Work out the finished part from the listing and answer in its coordinate system (mm). A direction names the side the tool comes from. Round coordinates to 2 decimals unless told otherwise and drop trailing zeros. Order: outer loops, then holes, each group sorted by start corner. A loop starts at its lowest first (then second) coordinate and runs counter-clockwise, first axis right, second up. Notation, with made-up numbers: (35.5, 21.5) - (64.5, 21.5) arc R24 ccw to (64.5, 46.5) - close; hole circle Ø4 at (-16, 33.25). An arc over 180 degrees is marked (long way). Use one line per item in the form item = value. Start each with the question number.
Q1. Which of the six approach directions +Z, -Z, +X, -X, +Y, -Y give full straight-line access (tool end or side, diameter ignored) to faces 1 (the cylindrical face through (77.496, 0.934, 0.986)), 2 (the flat face through (-33, 4, 2))?
Q2. The part is cut by section C-C on y = -36.5. Determine the outline of the cut face in (x, z).
Q3. The part is cut by section A-A on z = 2.85. State how many separate pieces and enclosed holes the cut face has, plus the area to 3 significant figures.
Q4. For a pull along Y with two mould halves and no side action, classify faces 3 (the cylindrical face through (-77.496, -0.934, 0.986)), 4 (the flat face through (30, -3, 4)), 5 (the flat face through (-33, -3, 2)) as +Y half, -Y half, draft (parallel to the pull), parting line (faces both ways), or undercut.
Q5. Given P1, Ø1.6, axis at y = -4, z = 2.5, coming from the +X side; P2, Ø0.6, axis at x = -15.5, z = 3.5, coming from the +Y side; P3, Ø2, axis at y = -41, z = 2.5, coming from the -X side; P4, Ø1.5, axis at x = -34, y = 4.5, coming from the +Z side, each flat-ended and moving along its own axis, determine where each tip first touches the part or whether it passes through.
Q6. The part is cut by section B-B on x = 43.5. Determine the outline of the cut face in (y, z), plus the area to 3 significant figures.
Q7. Find the intervals of material crossed by line 1 (Y direction, x = 1.5, z = 2.25); line 2 (Z direction, x = 58.5, y = 21); line 3 (X direction, y = 2, z = 0.6), in increasing order. Write a range as [from, to].
Autodesk Inventor part; units mm, degrees
ref_plane "YZ Plane" through (0, 0, 0) normal (1, 0, 0) x (0, 1, 0)
ref_plane "XZ Plane" through (0, 0, 0) normal (0, 1, 0) x (-1, 0, 0)
ref_plane "XY Plane" through (0, 0, 0) normal (0, 0, 1) x (1, 0, 0)
sketch "Sketch1" plane through (0, 0, 0) normal (0, 0, 1) x (1, 0, 0)
  line L0 (57.5, 62.5) -> (-57.5, 62.5)
  line L1 (-57.5, 62.5) -> (-57.5, -62.5)
  line L2 (-57.5, -62.5) -> (57.5, -62.5)
  line L3 (57.5, -62.5) -> (57.5, 62.5)
  line L4 (57.5, 62.5) -> (-57.5, -62.5) construction
  line L5 (-57.5, 62.5) -> (57.5, -62.5) construction
  line L6 (57.5, 0) -> (77.5, 0)
  line L7 (-57.5, 0) -> (-77.5, 0)
  arc A0 (-57.5, 62.5) -> (-57.5, -62.5) centre (30.1562, 0) ccw
  arc A1 (57.5, -62.5) -> (57.5, 62.5) centre (-30.1562, 0) ccw
  point P0 (0, 0)
  dimension "d0" = 115
  dimension "d1" = 125
  dimension "d2" = 20
  dimension "d3" = 20
extrude "Extrusion1" add sketch "Sketch1" along normal blind 2
sketch "Sketch2" plane through (0, 0, 2) normal (0, 0, 1) x (1, 0, 0)
  line L0 (-40.012, 8.7608) -> (40.012, 8.7608) construction
  line L1 (40.012, 8.7608) -> (40.012, -8.7608) construction
  line L2 (40.012, -8.7608) -> (-40.012, -8.7608) construction
  line L3 (-40.012, -8.7608) -> (-40.012, 8.7608) construction
  line L4 (-38.3346, 8.4789) -> (-33.3727, 8.4789)
  spline S0 degree 2 poles (-33.3727, 8.4789) (-30.2716, 8.4789) (-27.988, 5.8852) (-27.988, 4.1513) knots 0 0 0 1 2 2 2
  spline S1 degree 2 poles (-27.988, 4.1513) (-27.988, 3.0518) (-28.8197, 1.5435) (-29.7359, 0.7682) knots 0 0 0 1 2 2 2
  spline S2 degree 2 poles (-29.7359, 0.7682) (-27.9739, 0.148) (-26.5079, -2.2201) (-26.5079, -3.5593) knots 0 0 0 1 2 2 2
  spline S3 degree 2 poles (-26.5079, -3.5593) (-26.5079, -5.8993) (-29.7218, -8.5211) (-32.6397, -8.5211) knots 0 0 0 1 2 2 2
  line L5 (-32.6397, -8.5211) -> (-38.3346, -8.5211)
  line L6 (-38.3346, -8.5211) -> (-38.3346, 8.4789)
  line L7 (-34.6696, -0.9938) -> (-34.6696, -5.6737)
  line L8 (-34.6696, -5.6737) -> (-33.3445, -5.6737)
  spline S4 degree 2 poles (-33.3445, -5.6737) (-30.3279, -5.6737) (-30.3279, -3.4747) knots 0 0 0 1 1 1
  spline S5 degree 2 poles (-30.3279, -3.4747) (-30.3279, -2.2765) (-31.7939, -0.9938) (-33.1754, -0.9938) knots 0 0 0 1 2 2 2
  line L9 (-33.1754, -0.9938) -> (-34.6696, -0.9938)
  line L10 (-34.6696, 5.6314) -> (-34.6696, 1.8959)
  line L11 (-34.6696, 1.8959) -> (-33.8238, 1.8959)
  spline S6 degree 2 poles (-33.8238, 1.8959) (-32.8935, 1.8959) (-31.6248, 3.08) (-31.6248, 3.954) knots 0 0 0 1 2 2 2
  spline S7 degree 2 poles (-31.6248, 3.954) (-31.6248, 4.6588) (-32.8653, 5.6314) (-33.7956, 5.6314) knots 0 0 0 1 2 2 2
  line L12 (-33.7956, 5.6314) -> (-34.6696, 5.6314)
  line L13 (-24.2384, 8.7608) -> (-20.9258, 8.7608)
  line L14 (-20.9258, 8.7608) -> (-20.9258, -8.5211)
  line L15 (-20.9258, -8.5211) -> (-24.2384, -8.5211)
  line L16 (-24.2384, -8.5211) -> (-24.2384, 8.7608)
  line L17 (-17.5145, 2.5867) -> (-14.1455, 2.5867)
  line L18 (-14.1455, 2.5867) -> (-14.1455, -2.7558)
  spline S8 degree 2 poles (-14.1455, -2.7558) (-14.1455, -3.9117) (-12.9755, -5.4482) (-12.1157, -5.4482) knots 0 0 0 1 2 2 2
  spline S9 degree 2 poles (-12.1157, -5.4482) (-11.1994, -5.4482) (-9.9449, -3.954) (-9.9449, -2.8263) knots 0 0 0 1 2 2 2
  line L19 (-9.9449, -2.8263) -> (-9.9449, 2.5867)
  line L20 (-9.9449, 2.5867) -> (-6.5759, 2.5867)
  line L21 (-6.5759, 2.5867) -> (-6.5759, -3.8835)
  spline S10 degree 2 poles (-6.5759, -3.8835) (-6.5759, -5.9415) (-9.7193, -8.7326) (-12.0593, -8.7326) knots 0 0 0 1 2 2 2
  spline S11 degree 2 poles (-12.0593, -8.7326) (-14.5402, -8.7326) (-17.5145, -5.9415) (-17.5145, -3.6157) knots 0 0 0 1 2 2 2
  line L22 (-17.5145, -3.6157) -> (-17.5145, 2.5867)
  line L23 (6.9424, -3.7566) -> (-0.9938, -3.7566)
  spline S12 degree 2 poles (-0.9938, -3.7566) (-0.9233, -4.8279) (0.3595, -6.1671) (1.2052, -6.1671) knots 0 0 0 1 2 2 2
  spline S13 degree 2 poles (1.2052, -6.1671) (2.7417, -6.1671) (3.6016, -4.7857) knots 0 0 0 1 1 1
  line L24 (3.6016, -4.7857) -> (6.6464, -5.8006)
  spline S14 degree 2 poles (6.6464, -5.8006) (4.9548, -8.7608) (1.3744, -8.7608) knots 0 0 0 1 1 1
  spline S15 degree 2 poles (1.3744, -8.7608) (-1.2475, -8.7608) (-4.3628, -5.575) (-4.3628, -2.8827) knots 0 0 0 1 2 2 2
  spline S16 degree 2 poles (-4.3628, -2.8827) (-4.3628, -0.4581) (-1.0925, 2.8263) (1.3039, 2.8263) knots 0 0 0 1 2 2 2
  spline S17 degree 2 poles (1.3039, 2.8263) (3.7143, 2.8263) (6.9424, -0.6273) (6.9424, -3.221) knots 0 0 0 1 2 2 2
  line L25 (6.9424, -3.221) -> (6.9424, -3.7566)
  line L26 (-0.9656, -1.5294) -> (3.517, -1.5294)
  spline S18 degree 2 poles (3.517, -1.5294) (3.0518, 0.5568) (1.3744, 0.5568) knots 0 0 0 1 1 1
  spline S19 degree 2 poles (1.3744, 0.5568) (0.4158, 0.5568) (-0.8387, -0.5286) (-0.9656, -1.5294) knots 0 0 0 1 2 2 2
  line L27 (23.8719, 4.7857) -> (21.4332, 2.5021)
  spline S20 degree 2 poles (21.4332, 2.5021) (20.6721, 3.813) (18.4167, 5.124) (17.1903, 5.124) knots 0 0 0 1 2 2 2
  spline S21 degree 2 poles (17.1903, 5.124) (15.2027, 5.124) (12.2566, 2.0933) (12.2566, 0.0493) knots 0 0 0 1 2 2 2
  spline S22 degree 2 poles (12.2566, 0.0493) (12.2566, -2.1356) (15.1886, -5.1803) (17.2608, -5.1803) knots 0 0 0 1 2 2 2
  spline S23 degree 2 poles (17.2608, -5.1803) (18.3885, -5.1803) (20.4747, -4.0386) (21.109, -2.4739) knots 0 0 0 1 2 2 2
  line L28 (21.109, -2.4739) -> (17.0775, -2.4739)
  line L29 (17.0775, -2.4739) -> (17.0775, 0.8387)
  line L30 (17.0775, 0.8387) -> (24.9291, 0.8387)
  line L31 (24.9291, 0.8387) -> (24.9291, -1.3603)
  spline S24 degree 2 poles (24.9291, -1.3603) (24.9291, -3.0659) (22.6032, -6.9565) (18.7973, -8.7608) (16.852, -8.7608) knots 0 0 0 1 2 3 3 3
  spline S25 degree 2 poles (16.852, -8.7608) (13.3279, -8.7608) (8.493, -3.658) (8.493, 0.0916) knots 0 0 0 1 2 2 2
  spline S26 degree 2 poles (8.493, 0.0916) (8.493, 3.658) (13.483, 8.7044) (16.9789, 8.7044) knots 0 0 0 1 2 2 2
  spline S27 degree 2 poles (16.9789, 8.7044) (21.4614, 8.7044) (23.8719, 4.7857) knots 0 0 0 1 1 1
  spline S28 degree 2 poles (27.2127, -2.9813) (27.2127, -0.4017) (30.4971, 2.8545) (33.0767, 2.8545) knots 0 0 0 1 2 2 2
  spline S29 degree 2 poles (33.0767, 2.8545) (35.4731, 2.8545) (38.7152, -0.4722) (38.7152, -2.9391) knots 0 0 0 1 2 2 2
  spline S30 degree 2 poles (38.7152, -2.9391) (38.7152, -5.4482) (35.4731, -8.7608) (33.0203, -8.7608) knots 0 0 0 1 2 2 2
  spline S31 degree 2 poles (33.0203, -8.7608) (30.2716, -8.7608) (27.2127, -5.2508) (27.2127, -2.9813) knots 0 0 0 1 2 2 2
  spline S32 degree 2 poles (35.459, -2.9813) (35.459, -1.8536) (33.9789, -0.1762) (32.9921, -0.1762) knots 0 0 0 1 2 2 2
  spline S33 degree 2 poles (32.9921, -0.1762) (31.9772, -0.1762) (30.4971, -1.755) (30.4971, -2.8545) knots 0 0 0 1 2 2 2
  spline S34 degree 2 poles (30.4971, -2.8545) (30.4971, -4.0667) (31.9631, -5.7442) (32.9921, -5.7442) knots 0 0 0 1 2 2 2
  spline S35 degree 2 poles (32.9921, -5.7442) (33.9789, -5.7442) (35.459, -4.0949) (35.459, -2.9813) knots 0 0 0 1 2 2 2
  point P0 (0, 0)
extrude "Extrusion2" add sketch "Sketch2" along normal blind 2
sketch "Sketch3" plane through (-38.3346, -8.5211, 2) normal (-1, 0, 0) x (0, 0, 1)
  point P0 (-2, 8.5211)
properties part number "BlueGo"
Found:
q1.face_1 = +Z, -Z, +X
q1.face_2 = +Z
q2.outline = (-71.12, 0) - (71.12, 0) - (71.12, 2) - (-71.12, 2) - close
q3.separate_pieces = 6
q3.enclosed_holes = 4
q3.area = 613 mm²
q4.face_3 = parting line
q4.face_4 = draft
q4.face_5 = undercut
q5.P1 = 77.45
q5.P2 = 2.59
q5.P3 = -69.74
q5.P4 = 4
q6.outline = (-62.5, 0) - (62.5, 0) - (62.5, 2) - (-62.5, 2) - close
q6.area = 250 mm²
q7.line_1 = [-8.76, -6.15], [-3.76, -1.53], [0.55, 2.82]
q7.line_2 = [0, 2]
q7.line_3 = [-77.48, 77.48]
